The model under review builds one solid part; all positions refer to its coordinate system, in mm. Round coordinates to 2 decimals unless told otherwise and drop trailing zeros. Write each loop counter-clockwise with the first axis right and the second up, starting at its lowest first coordinate (ties: lowest second). Pieces come first, ordered by that corner, then holes.
Item 1: Clearance check with flat-ended pins moving along their axes: pin 1 Ø3 at (x, z) = (-1, 0.5) entering from -Y; pin 2 Ø1 at (y, z) = (-2.5, -1.5) entering from -X. State where each tip first meets the part, or that it passes through.
Item 2: Add section B-B (x = 0). Give the boundary of the cut face in (y, z).
Item 3: To check wall thickness, follow L1, parallel to Y at x = 0.75, z = -0.25. State the ranges of the line that lie inside material, in increasing order.
Item 4: Add section A-A (z = -1.5). Give the boundary of the cut face in (x, y), plus the area to 3 significant figures.
```python
from build123d import *

# Parameters (mm, degrees)
SKETCH1_W           = 6.223
SKETCH1_H           = 6.223
BOSS_EXTRUDE1_DEPTH = 3.81
SKETCH2_R           = 0.3175
BOSS_EXTRUDE2_DEPTH = 8.89


with BuildPart() as part:
    # Sketch1 → Boss-Extrude1 (new body)
    with BuildSketch(Plane(origin=(0, 0, 0), x_dir=(1, 0, 0), z_dir=(0, 1, 0))):
        Rectangle(SKETCH1_W, SKETCH1_H)
    extrude(amount=BOSS_EXTRUDE1_DEPTH)

    # Sketch2 → Boss-Extrude2 (add)
    with BuildSketch(Plane.XZ):
        with Locations(Location((-2.794, 0, 0), (0, 0, 180))):
            Circle(SKETCH2_R)
        with Locations((2.794, 0)):
            Circle(SKETCH2_R)
    extrude(amount=BOSS_EXTRUDE2_DEPTH)


solid = part.part
```
Numbers:
1. pin 1: stops at y = 0
1. pin 2: passes through
2. outline: (0, -3.11) - (3.81, -3.11) - (3.81, 3.11) - (0, 3.11) - close
3. L1: y = 0 to 3.81
4. outline: (-3.11, 0) - (3.11, 0) - (3.11, 3.81) - (-3.11, 3.81) - close
4. area: 23.7 mm2
